Autodesk Inventor part; units mm, degrees
ref_plane "YZ Plane" through (0, 0, 0) normal (1, 0, 0) x (0, 1, 0)
ref_plane "XZ Plane" through (0, 0, 0) normal (0, 1, 0) x (-1, 0, 0)
ref_plane "XY Plane" through (0, 0, 0) normal (0, 0, 1) x (1, 0, 0)
sketch "Sketch1" plane through (0, 0, 0) normal (0, 0, 1) x (1, 0, 0)
  line L0 (0, 1490) -> (-178.9061, 1490)
  line L1 (-178.9061, 1490) -> (-178.9061, 0)
  line L2 (-178.9061, 0) -> (0, 0)
  line L3 (0, 0) -> (0, 1490)
  line L4 (-178.9061, 100) -> (-66, 100)
  line L5 (-66, 100) -> (-66, 105)
  line L6 (-66, 105) -> (-178.9061, 105)
  line L7 (-178.9061, 105) -> (-178.9061, 100)
  line L8 (-178.9061, 596.6667) -> (-66, 596.6667)
  line L9 (-66, 596.6667) -> (-66, 601.6667)
  line L10 (-66, 601.6667) -> (-178.9061, 601.6667)
  line L11 (-178.9061, 601.6667) -> (-178.9061, 596.6667)
  line L12 (-178.9061, 1093.3333) -> (-66, 1093.3333)
  line L13 (-66, 1093.3333) -> (-66, 1098.3333)
  line L14 (-66, 1098.3333) -> (-178.9061, 1098.3333)
  line L15 (-178.9061, 1098.3333) -> (-178.9061, 1093.3333)
  circle A0 centre (-178.9061, 1335) radius 30
  point P0 (-178.9061, 1098.3333)
  point P1 (-178.9061, 1093.3333)
  point P2 (-178.9061, 596.6667)
  point P3 (-178.9061, 105)
  point P4 (-178.9061, 1365)
  point P5 (-178.9061, 1305)
  dimension "d0" = 1490
  dimension "d1" = 178.9061
  dimension "d2" = 5
  dimension "d4" = 100
  dimension "d7" = 496.6667
  dimension "d23" = 66
  dimension "d29" = 60
  dimension "d30" = 1335
extrude "Plate1" add sketch "Sketch1" along normal blind 4 contours L3 L2 L1 L4 L5 L6 L8 L9 L10 L12 L13 L14 A0 L0
chamfer "Corner Chamfer1" distance 3 angle 45 6 edges at (-178.9061, 100, 2) (-178.9061, 105, 2) (-178.9061, 596.6667, 2) (-178.9061, 601.6667, 2) (-178.9061, 1098.3333, 2) (-178.9061, 1093.3333, 2)
equation "\"d0\" = Стрингер_длина"
equation "\"d1\" = стрингер_глубина_2"
equation "\"d2\" = паз_под_стрингер_толщина"
equation "\"d7\" = Шаг_шпангоутов"
equation "\"d23\" = паз_под_стрингер_глубина - Thickness"
equation "\"d29\" = 2 * радиус_выреза_под_сварку"
equation "\"d12\" = Thickness"
equation "\"BendRadius\" = Thickness"
equation "\"BendReliefWidth\" = Thickness"
equation "\"BendReliefDepth\" = 0.5 * Thickness"
equation "\"CornerReliefSize\" = 4 * Thickness"
equation "\"MinimumRemnant\" = 2 * Thickness"
equation "\"TransitionRadius\" = BendRadius"
equation "\"JacobiRadiusSize\" = BendRadius"
equation "\"GapSize\" = Thickness"
properties part number "0414 GBK stringer C2" material "Steel"
Source: CAD feature listing. Evaluate the final solid. Frame: model axes, mm. Give positions to 0.01 mm unless a question says otherwise; leave off trailing zeros. Write each loop counter-clockwise with the first axis right and the second up, starting at its lowest first coordinate (ties: lowest second). Pieces come first, ordered by that corner, then holes. Notation, with made-up numbers: M 58.25,-16 L 112.25,-16 A19 cw 112.25,2 Z; hole C 68,-29 d2. An arc over 180 degrees is marked long. Return JSON: item names as keys, results as strings. Group by question number.
1) First-contact query: pin 1 Ø1.2 at (y, z) = (103.5, 1.5) entering from -X. Flat tip, straight axial feed; report the tip coordinate or a pass-through.
2) Cut plane A-A, the plane y = 1335. Output: boundary loops of the cut face in (x, z).
3) Ray query, L1, parallel to Y at x = -115, z = 3.65; L2, parallel to Y at x = -168, z = 0.6. Return the intervals inside material, ascending.
4) Draft query along Y for faces 1 (the face through (-148.913, 1335.66, 1.972)), 2 (the face through (-91, 755, 4)). Return one class per face: released by +Y, released by -Y, zero draft, split by the parting line, or undercut.
Data:
{
 "1": {"pin 1": "stops at x = -66"},
 "2": {"outline": "M -148.91,0 L 0,0 L 0,4 L -148.91,4 Z"},
 "3": {"L1": "y = 0 to 100, 105 to 596.67, 601.67 to 1093.33, 1098.33 to 1490", "L2": "y = 0 to 100, 105 to 596.67, 601.67 to 1093.33, 1098.33 to 1307.05, 1362.95 to 1490"},
 "4": {"face 1": "undercut", "face 2": "zero draft"}
}
